```python
from build123d import *

# Parameters (mm, degrees)
BOSS_EXTRUDE2_DEPTH = 3.175
SKETCH3_R           = 12.1285
CUT_EXTRUDE2_DEPTH  = 92.247975457
SKETCH4_R           = 38.1
CUT_EXTRUDE3_DEPTH  = 92.247975457
CUT_EXTRUDE6_DEPTH  = 92.247975457
BOSS_EXTRUDE3_DEPTH = 3.175
SKETCH12_R          = 1.143
CUT_EXTRUDE9_DEPTH  = 97.166400707
SKETCH13_R          = 1.651
CUT_EXTRUDE10_DEPTH = 55.88
SKETCH14_R          = 3.175
CUT_EXTRUDE11_DEPTH = 129.184225337


with BuildPart() as part:
    # Sketch1 → Boss-Extrude2 (new body)
    with BuildSketch(Plane.XY):
        with BuildLine():
            Line((-60.107370596, 33.02), (-55.027370596, 33.02))
            Line((-55.027370596, 33.02), (-55.027370596, -33.02))
            Line((-55.027370596, -33.02), (-60.107370596, -33.02))
            ThreePointArc((-60.107370596, -33.02), (0, -68.58), (60.107370596, -33.02))
            Line((60.107370596, -33.02), (55.027370596, -33.02))
            Line((55.027370596, -33.02), (55.027370596, 33.02))
            Line((55.027370596, 33.02), (60.107370596, 33.02))
            ThreePointArc((60.107370596, 33.02), (0, 68.58), (-60.107370596, 33.02))
        make_face()
    extrude(amount=BOSS_EXTRUDE2_DEPTH)

    # Sketch3 → Cut-Extrude2 (cut, through all)
    with BuildSketch(Plane(origin=(0, 0, 0), x_dir=(-1, 0, 0), z_dir=(0, 0, -1))):
        with Locations((14.224, -34.29)):
            Circle(SKETCH3_R)
        with Locations(Location((14.224, 34.29, 0), (0, 0, 180))):
            Circle(SKETCH3_R)
        with Locations((-14.224, 34.29)):
            Circle(SKETCH3_R)
        with Locations(Location((-14.224, -34.29, 0), (0, 0, 180))):
            Circle(SKETCH3_R)
    extrude(amount=-CUT_EXTRUDE2_DEPTH, mode=Mode.SUBTRACT)

    # Sketch4 → Cut-Extrude3 (cut, through all)
    with BuildSketch(Plane(origin=(0, 0, 0), x_dir=(-1, 0, 0), z_dir=(0, 0, -1))):
        with Locations((0, -86.312058398)):
            Circle(SKETCH4_R)
    extrude(amount=-CUT_EXTRUDE3_DEPTH, mode=Mode.SUBTRACT)

    # Sketch5 → Cut-Extrude6 (cut, through all)
    with BuildSketch(Plane(origin=(0, 0, 0), x_dir=(-1, 0, 0), z_dir=(0, 0, -1))):
        with BuildLine():
            Line((10.776307345, -10.776307345), (19.793695097, -19.793695097))
            Line((19.793695097, -19.793695097), (30.704765274, -22.71730754))
            Line((30.704765274, -22.71730754), (30.704765274, -34.85110441))
            Line((30.704765274, -34.85110441), (29.410338797, -36.145530887))
            Line((29.410338797, -36.145530887), (45.008715274, -51.743907365))
            ThreePointArc((45.008715274, -51.743907365), (46.779291091, -50.148921474), (48.493383054, -48.493383054))
            Line((48.493383054, -48.493383054), (33.244765274, -33.244765274))
            Line((33.244765274, -33.244765274), (33.244765274, -20.76829699))
            Line((33.244765274, -20.76829699), (21.108495846, -17.516393398))
            Line((21.108495846, -17.516393398), (12.421633561, -8.829531113))
            Line((12.421633561, -8.829531113), (10.625582337, -10.625582337))
            Line((10.625582337, -10.625582337), (10.776307345, -10.776307345))
        make_face()
        with BuildLine():
            Line((-10.776307345, -10.776307345), (-10.625582337, -10.625582337))
            Line((-10.625582337, -10.625582337), (-12.421633561, -8.829531113))
            Line((-12.421633561, -8.829531113), (-21.108495846, -17.516393398))
            Line((-21.108495846, -17.516393398), (-33.244765274, -20.76829699))
            Line((-33.244765274, -20.76829699), (-33.244765274, -33.244765274))
            Line((-33.244765274, -33.244765274), (-48.493383054, -48.493383054))
            ThreePointArc((-48.493383054, -48.493383054), (-46.779291091, -50.148921474), (-45.008715274, -51.743907365))
            Line((-45.008715274, -51.743907365), (-29.410338797, -36.145530887))
            Line((-29.410338797, -36.145530887), (-30.704765274, -34.85110441))
            Line((-30.704765274, -34.85110441), (-30.704765274, -22.71730754))
            Line((-30.704765274, -22.71730754), (-19.793695097, -19.793695097))
            Line((-19.793695097, -19.793695097), (-10.776307345, -10.776307345))
        make_face()
        with BuildLine():
            Line((-10.776307345, 10.776307345), (-19.793695097, 19.793695097))
            Line((-19.793695097, 19.793695097), (-30.704765274, 22.71730754))
            Line((-30.704765274, 22.71730754), (-30.704765274, 34.85110441))
            Line((-30.704765274, 34.85110441), (-29.410338797, 36.145530887))
            Line((-29.410338797, 36.145530887), (-45.008715274, 51.743907365))
            ThreePointArc((-45.008715274, 51.743907365), (-46.779291091, 50.148921474), (-48.493383054, 48.493383054))
            Line((-48.493383054, 48.493383054), (-33.244765274, 33.244765274))
            Line((-33.244765274, 33.244765274), (-33.244765274, 20.76829699))
            Line((-33.244765274, 20.76829699), (-21.108495846, 17.516393398))
            Line((-21.108495846, 17.516393398), (-12.421633561, 8.829531113))
            Line((-12.421633561, 8.829531113), (-10.625582337, 10.625582337))
            Line((-10.625582337, 10.625582337), (-10.776307345, 10.776307345))
        make_face()
        with BuildLine():
            ThreePointArc((48.493383054, 48.493383054), (46.779291091, 50.148921474), (45.008715274, 51.743907365))
            Line((45.008715274, 51.743907365), (29.410338797, 36.145530887))
            Line((29.410338797, 36.145530887), (30.704765274, 34.85110441))
            Line((30.704765274, 34.85110441), (30.704765274, 22.71730754))
            Line((30.704765274, 22.71730754), (19.793695097, 19.793695097))
            Line((19.793695097, 19.793695097), (10.776307345, 10.776307345))
            Line((10.776307345, 10.776307345), (10.625582337, 10.625582337))
            Line((10.625582337, 10.625582337), (12.421633561, 8.829531113))
            Line((12.421633561, 8.829531113), (21.108495846, 17.516393398))
            Line((21.108495846, 17.516393398), (33.244765274, 20.76829699))
            Line((33.244765274, 20.76829699), (33.244765274, 33.244765274))
            Line((33.244765274, 33.244765274), (48.493383054, 48.493383054))
        make_face()
    extrude(amount=-CUT_EXTRUDE6_DEPTH, mode=Mode.SUBTRACT)

    # Sketch9 → Boss-Extrude3 (add)
    with BuildSketch(Plane(origin=(0, 0, 0), x_dir=(-1, 0, 0), z_dir=(0, 0, -1))):
        with BuildLine():
            Line((12.7, 67.39381574), (0, 75))
            Line((0, 75), (-12.7, 67.39381574))
            ThreePointArc((-12.7, 67.39381574), (0, 68.58), (12.7, 67.39381574))
        make_face()
    extrude(amount=-BOSS_EXTRUDE3_DEPTH)

    # Sketch12 → Cut-Extrude9 (cut, through all)
    with BuildSketch(Plane(origin=(0, 0, 0), x_dir=(-1, 0, 0), z_dir=(0, 0, -1))):
        with Locations((6.731, 62.23)):
            Circle(SKETCH12_R)
        with Locations((-6.731, 62.23)):
            Circle(SKETCH12_R)
    extrude(amount=-CUT_EXTRUDE9_DEPTH, mode=Mode.SUBTRACT)

    # Sketch13 → Cut-Extrude10 (cut)
    with BuildSketch(Plane(origin=(30.092005081, 4.08352975, 15.875), x_dir=(1, 0, 0), z_dir=(0, 0, 1))):
        with Locations((-54.476005081, -49.80352975)):
            Circle(SKETCH13_R)
        with Locations((-54.476005081, 41.63647025)):
            Circle(SKETCH13_R)
        with Locations((-5.708005081, -49.80352975)):
            Circle(SKETCH13_R)
        with Locations((-5.708005081, 41.63647025)):
            Circle(SKETCH13_R)
    extrude(amount=-CUT_EXTRUDE10_DEPTH, mode=Mode.SUBTRACT)

    # Sketch14 → Cut-Extrude11 (cut, through all)
    with BuildSketch(Plane(origin=(30.092005081, 4.08352975, -53.975), x_dir=(-1, 0, 0), z_dir=(0, 0, -1))):
        with Locations(Location((-13.087994919, 21.31647025, 0), (0, 0, 180))):
            Circle(SKETCH14_R)
        with Locations((73.272005081, 21.31647025)):
            Circle(SKETCH14_R)
        with Locations((30.092005081, 21.31647025)):
            Circle(SKETCH14_R)
        with Locations(Location((73.272005081, -29.48352975, 0), (0, 0, 180))):
            Circle(SKETCH14_R)
        with Locations(Location((30.092005081, -29.48352975, 0), (0, 0, 180))):
            Circle(SKETCH14_R)
        with Locations((-13.087994919, -29.48352975)):
            Circle(SKETCH14_R)
    extrude(amount=-CUT_EXTRUDE11_DEPTH, mode=Mode.SUBTRACT)


solid = part.part
```
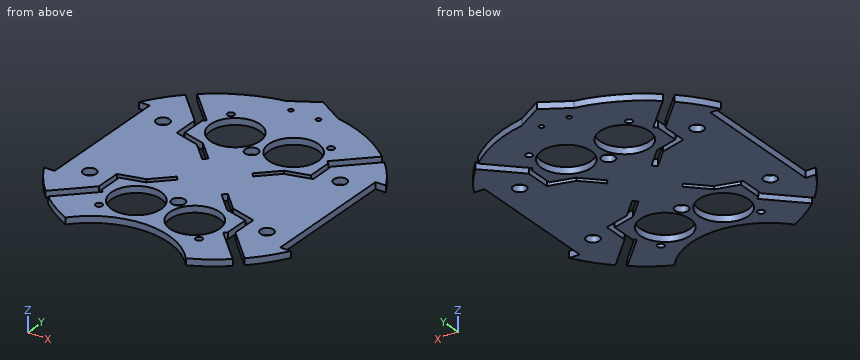
CAD build for the part. Positions are in the model's coordinates, mm. Coordinates: 2 decimals unless noted, no trailing zeros. Order: outer loops, then holes, each group sorted by start corner. A loop starts at its lowest first (then second) coordinate and runs counter-clockwise, first axis right, second up. Notation, with made-up numbers: (52.25, 89) - (105.25, 89) arc R20 cw to (105.25, 106) - close; hole circle Ø9 at (-32, 31.5). An arc over 180 degrees is marked (long way). Use a Markdown table: item, result. Add a question column.
(1) Saw through at A-A (x = 43.18). Give the cut face in (y, z) (3 decimals), then the cut area to 3 significant figures.
(2) Drill centre lines: line 1 along Y through (x, z) = (0, 1.3) (3 decimals); line 2 along Y through (x, z) = (43, 1.6); line 3 along Y through (x, z) = (27, 2.95). Where is each one in solid material? Low to high. Write a range as [from, to].
(3) Saw through at D-D (y = 6). Give the cut face in (x, z) (3 decimals), then the cut area to 3 significant figures.
(4) Flat gauge pin, fed straight in: pin 1 (1.5 mm diameter, centred on y = 11, z = 2, fed in from +X). Where does the tip first touch, or does it go through?
(5) Saw through at B-B (y = -25.4). Count the separate pieces of the cut face and the enclosed holes in it, then the cut area to 3 significant figures.
Solved:
| question | item | result |
|---|---|---|
| 1 | outline | (-53.279, 0) - (-49.915, 0) - (-49.915, 3.175) - (-53.279, 3.175) - close; (-43.18, 0) - (-28.575, 0) - (-28.575, 3.175) - (-43.18, 3.175) - close; (-22.225, 0) - (22.225, 0) - (22.225, 3.175) - (-22.225, 3.175) - close; (28.575, 0) - (43.18, 0) - (43.18, 3.175) - (28.575, 3.175) - close; (49.915, 0) - (53.279, 0) - (53.279, 3.175) - (49.915, 3.175) - close |
| 1 | area | 255 mm² |
| 2 | line 1 | y = [-48.212, -28.575], [-22.225, 22.225], [28.575, 75] |
| 2 | line 2 | y = [-53.42, -49.74], [-43, -28.57], [-22.23, 22.23], [28.57, 43], [49.74, 53.42] |
| 2 | line 3 | y = [-59.43, -21.72], [-19.1, 19.1], [21.72, 63.04] |
| 3 | outline | (-55.027, 0) - (55.027, 0) - (55.027, 3.175) - (-55.027, 3.175) - close |
| 3 | area | 349 mm² |
| 4 | pin 1 | stops at x = 55.03 |
| 5 | separate pieces | 8 |
| 5 | enclosed holes | 0 |
| 5 | area | 168 mm² |
